from build123d import *

# Parameters (mm, degrees)
BOSS_EXTRUDE1_DEPTH = 50.8
SKETCH2_R           = 3.175
CUT_EXTRUDE2_DEPTH  = 123.36896502


with BuildPart() as part:
    # Sketch1 → Boss-Extrude1 (new body)
    with BuildSketch(Plane(origin=(0, 0, 0), x_dir=(1, 0, 0), z_dir=(0, 1, 0))):
        with BuildLine():
            Line((0, 101.6), (2.54, 101.6))
            Line((2.54, 101.6), (2.54, 5.08))
            ThreePointArc((2.54, 5.08), (3.283948776, 3.283948776), (5.08, 2.54))
            Line((5.08, 2.54), (45.72, 2.54))
            ThreePointArc((45.72, 2.54), (47.516051224, 3.283948776), (48.26, 5.08))
            Line((48.26, 5.08), (48.26, 101.6))
            Line((48.26, 101.6), (50.8, 101.6))
            Line((50.8, 101.6), (50.8, 5.08))
            ThreePointArc((50.8, 5.08), (49.312102448, 1.487897552), (45.72, 0))
            Line((45.72, 0), (5.08, 0))
            ThreePointArc((5.08, 0), (1.487897552, 1.487897552), (0, 5.08))
            Line((0, 5.08), (0, 101.6))
        make_face()
    extrude(amount=BOSS_EXTRUDE1_DEPTH)

    # Sketch2 → Cut-Extrude2 (cut, through all)
    with BuildSketch(Plane(origin=(0, 0, -2.54), x_dir=(-1, 0, 0), z_dir=(0, 0, -1))):
        with Locations((-34.925, 25.4)):
            Circle(SKETCH2_R)
        with Locations((-25.4, 34.925)):
            Circle(SKETCH2_R)
        with Locations((-15.875, 25.4)):
            Circle(SKETCH2_R)
        with Locations((-25.4, 15.875)):
            Circle(SKETCH2_R)
    extrude(amount=-CUT_EXTRUDE2_DEPTH, mode=Mode.SUBTRACT)


solid = part.part
The listing builds one solid part. Answer for the finished solid, in the listing's coordinates (mm). A direction names the side the tool comes from. Coordinates: 2 decimals unless noted, no trailing zeros. Write each loop counter-clockwise with the first axis right and the second up, starting at its lowest first coordinate (ties: lowest second). Pieces come first, ordered by that corner, then holes. Notation, with made-up numbers: (41.25, 34.5) - (98.25, 34.5) arc R13 ccw to (98.25, 44.5) - close; hole circle Ø9 at (43.5, -39). An arc over 180 degrees is marked (long way). Return JSON: item names as keys, results as strings.
1. The part is cut by section A-A on x = 25.4. Determine the outline of the cut face in (y, z), then the cut area to 3 significant figures.
Final values:
{"outline": "(0, -2.54) - (12.7, -2.54) - (12.7, 0) - (0, 0) - close; (19.05, -2.54) - (31.75, -2.54) - (31.75, 0) - (19.05, 0) - close; (38.1, -2.54) - (50.8, -2.54) - (50.8, 0) - (38.1, 0) - close", "area": "96.8 mm^2"}
2. This flat-tipped pin is pushed along its axis until it touches: pin 1 Ø1.5 at (x, y) = (17, 36) entering from -Z. Where does it stop, or does it pass through?
Final values:
{"pin 1": "z = -2.54"}
3. For a pull along X with two mould halves and no side action, classify faces 3 (the face through (1.528, 25.044, -1.449)), 4 (the face through (1, 50.8, -36)), 5 (the face through (16.288, 28.548, -1.288)) as +X half, -X half, draft (parallel to the pull), parting line (faces both ways), or undercut.
Final values:
{"face 3": "-X half", "face 4": "draft", "face 5": "undercut"}
4. The part is cut by section B-B on y = 25.4. Determine the outline of the cut face in (x, z).
Final values:
{"outline": "(0, -101.6) - (2.54, -101.6) - (2.54, -5.08) arc R2.54 cw to (5.08, -2.54) - (12.7, -2.54) - (12.7, 0) - (5.08, 0) arc R5.08 ccw to (0, -5.08) - close; (19.05, -2.54) - (31.75, -2.54) - (31.75, 0) - (19.05, 0) - close; (38.1, -2.54) - (45.72, -2.54) arc R2.54 cw to (48.26, -5.08) - (48.26, -101.6) - (50.8, -101.6) - (50.8, -5.08) arc R5.08 ccw to (45.72, 0) - (38.1, 0) - close"}
5. The part is cut by section D-D on x = 34. Determine the outline of the cut face in (y, z).
Final values:
{"outline": "(0, -2.54) - (22.36, -2.54) - (22.36, 0) - (0, 0) - close; (28.44, -2.54) - (50.8, -2.54) - (50.8, 0) - (28.44, 0) - close"}
6. Which of the six approach directions +Z, -Z, +X, -X, +Y, -Y give full straight-line access (tool end or side, diameter ignored) to faces 1 (the face through (0, 25, -53)), 2 (the face through (3.264, 25.044, -3.304))?
Final values:
{"face 1": "+Z, -Z, -X, +Y, -Y", "face 2": "-Z, +Y, -Y"}
7. Consider line 1 along Y through (x, z) = (25, -2); line 2 along X through (y, z) = (2, -90.5); line 3 along Z through (x, y) = (40.5, 13). Determine where each line is inside the solid, lowest interval first.
Final values:
{"line 1": "0 to 12.73, 19.02 to 31.78, 38.07 to 50.8", "line 2": "0 to 2.54, 48.26 to 50.8", "line 3": "-2.54 to 0"}
8. The part is cut by section C-C on z = -58.5. Determine the outline of the cut face in (x, y).
Final values:
{"outline": "(0, 0) - (2.54, 0) - (2.54, 50.8) - (0, 50.8) - close; (48.26, 0) - (50.8, 0) - (50.8, 50.8) - (48.26, 50.8) - close"}
